The model under review builds one solid part; all positions refer to its coordinate system, in mm. A direction names the side the tool comes from. Coordinates: 2 decimals unless noted, no trailing zeros. Write each loop counter-clockwise with the first axis right and the second up, starting at its lowest first coordinate (ties: lowest second). Pieces come first, ordered by that corner, then holes. Notation, with made-up numbers: (2, -6) -> (11, -6) arc R17 ccw to (11, 9) -> close; hole circle Ø2 at (52.5, -16). An arc over 180 degrees is marked (long way). Put each result on its own line as item: value. Start each with the question number.
from build123d import *

# Parameters (mm, degrees)
BOSS_EXTRUDE1_DEPTH = 50
SKETCH2_R           = 9
CUT_EXTRUDE1_DEPTH  = 50
SKETCH4_R           = 12.5
CUT_EXTRUDE2_DEPTH  = 35
SKETCH7_R           = 35
CUT_EXTRUDE3_DEPTH  = 20
FILLET1_R           = 3
SKETCH8_R           = 50
SKETCH8_R_2         = 43
CUT_EXTRUDE4_DEPTH  = 10
CUT_EXTRUDE5_DEPTH  = 20


with BuildPart() as part:
    # Sketch1 → Boss-Extrude1 (new body)
    with BuildSketch(Plane(origin=(0, 0, 0), x_dir=(1, 0, 0), z_dir=(0, 1, 0))):
        with BuildLine():
            Line((-105, -90), (105, -90))
            ThreePointArc((105, -90), (119.142135624, -84.142135624), (125, -70))
            Line((125, -70), (125, 70))
            ThreePointArc((125, 70), (119.142135624, 84.142135624), (105, 90))
            Line((105, 90), (-105, 90))
            ThreePointArc((-105, 90), (-119.142135624, 84.142135624), (-125, 70))
            Line((-125, 70), (-125, -70))
            ThreePointArc((-125, -70), (-119.142135624, -84.142135624), (-105, -90))
        make_face()
    extrude(amount=BOSS_EXTRUDE1_DEPTH)

    # Sketch2 → Cut-Extrude1 (cut)
    with BuildSketch(Plane(origin=(0, 50, 0), x_dir=(1, 0, 0), z_dir=(0, 1, 0))):
        with Locations((-100, -70)):
            Circle(SKETCH2_R)
        with Locations((-33, -70)):
            Circle(SKETCH2_R)
        with Locations((33, -70)):
            Circle(SKETCH2_R)
        with Locations((100, -70)):
            Circle(SKETCH2_R)
        with Locations((100, 70)):
            Circle(SKETCH2_R)
        with Locations((33, 70)):
            Circle(SKETCH2_R)
        with Locations((-33, 70)):
            Circle(SKETCH2_R)
        with Locations((-100, 70)):
            Circle(SKETCH2_R)
    extrude(amount=-CUT_EXTRUDE1_DEPTH, mode=Mode.SUBTRACT)

    # Sketch4 → Cut-Extrude2 (cut)
    with BuildSketch(Plane(origin=(0, 35, 0), x_dir=(1, 0, 0), z_dir=(0, 1, 0))):
        with Locations((-100, -70)):
            Circle(SKETCH4_R)
        with Locations((-33, -70)):
            Circle(SKETCH4_R)
        with Locations((33, -70)):
            Circle(SKETCH4_R)
        with Locations((100, -70)):
            Circle(SKETCH4_R)
        with Locations((100, 70)):
            Circle(SKETCH4_R)
        with Locations((33, 70)):
            Circle(SKETCH4_R)
        with Locations((-33, 70)):
            Circle(SKETCH4_R)
        with Locations((-100, 70)):
            Circle(SKETCH4_R)
    extrude(amount=-CUT_EXTRUDE2_DEPTH, mode=Mode.SUBTRACT)

    # Sketch7 → Cut-Extrude3 (cut)
    with BuildSketch(Plane(origin=(0, 50, 0), x_dir=(1, 0, 0), z_dir=(0, 1, 0))):
        with Locations((-65, 0)):
            Circle(SKETCH7_R)
        with Locations((65, 0)):
            Circle(SKETCH7_R)
    extrude(amount=-CUT_EXTRUDE3_DEPTH, mode=Mode.SUBTRACT)

    # Fillet1
    fillet1_edges = [part.edges().sort_by_distance(p)[0] for p in [
        (-100, 30, 0),
        (30, 30, 0),
    ]]
    fillet(fillet1_edges, radius=FILLET1_R)

    # Sketch8 → Cut-Extrude4 (cut)
    with BuildSketch(Plane(origin=(0, 50, 0), x_dir=(1, 0, 0), z_dir=(0, 1, 0))):
        with Locations((-65, 0)):
            Circle(SKETCH8_R)
        with Locations((-65, 0)):
            Circle(SKETCH8_R_2, mode=Mode.SUBTRACT)
        with Locations((65, 0)):
            Circle(SKETCH8_R)
        with Locations((65, 0)):
            Circle(SKETCH8_R_2, mode=Mode.SUBTRACT)
    extrude(amount=-CUT_EXTRUDE4_DEPTH, mode=Mode.SUBTRACT)

    # Sketch9 → Cut-Extrude5 (cut)
    with BuildSketch(Plane(origin=(0, 50, 0), x_dir=(1, 0, 0), z_dir=(0, 1, 0))):
        with BuildLine():
            Line((-53.124611797, -79), (-79.875388203, -79))
            ThreePointArc((-79.875388203, -79), (-82.28073938, -77.792842914), (-82.750332745, -75.142857143))
            ThreePointArc((-82.750332745, -75.142857143), (-82.776149203, -64.771332509), (-88.520347372, -56.135744681))
            ThreePointArc((-88.520347372, -56.135744681), (-89.185331801, -52.291224502), (-85.489464765, -51.040981903))
            ThreePointArc((-85.489464765, -51.040981903), (-67.418125523, -54.946816732), (-49.07353502, -52.643591379))
            ThreePointArc((-49.07353502, -52.643591379), (-45.649930196, -53.942627335), (-46.032701785, -57.584337142))
            ThreePointArc((-46.032701785, -57.584337142), (-50.502310556, -65.796534146), (-50.249667255, -75.142857143))
            ThreePointArc((-50.249667255, -75.142857143), (-50.71926062, -77.792842914), (-53.124611797, -79))
        make_face()
        with BuildLine():
            Line((53.124611797, 79), (79.875388203, 79))
            ThreePointArc((79.875388203, 79), (82.28073938, 77.792842914), (82.750332745, 75.142857143))
            ThreePointArc((82.750332745, 75.142857143), (82.776149203, 64.771332509), (88.520347372, 56.135744681))
            ThreePointArc((88.520347372, 56.135744681), (89.185331801, 52.291224502), (85.489464765, 51.040981903))
            ThreePointArc((85.489464765, 51.040981903), (67.418125523, 54.946816732), (49.07353502, 52.643591379))
            ThreePointArc((49.07353502, 52.643591379), (45.649930196, 53.942627335), (46.032701785, 57.584337142))
            ThreePointArc((46.032701785, 57.584337142), (50.502310556, 65.796534146), (50.249667255, 75.142857143))
            ThreePointArc((50.249667255, 75.142857143), (50.71926062, 77.792842914), (53.124611797, 79))
        make_face()
        with BuildLine():
            Line((-53.124611797, 79), (-79.875388203, 79))
            ThreePointArc((-79.875388203, 79), (-82.28073938, 77.792842914), (-82.750332745, 75.142857143))
            ThreePointArc((-82.750332745, 75.142857143), (-82.776149203, 64.771332509), (-88.520347372, 56.135744681))
            ThreePointArc((-88.520347372, 56.135744681), (-89.185331801, 52.291224502), (-85.489464765, 51.040981903))
            ThreePointArc((-85.489464765, 51.040981903), (-67.418125523, 54.946816732), (-49.07353502, 52.643591379))
            ThreePointArc((-49.07353502, 52.643591379), (-45.649930196, 53.942627335), (-46.032701785, 57.584337142))
            ThreePointArc((-46.032701785, 57.584337142), (-50.502310556, 65.796534146), (-50.249667255, 75.142857143))
            ThreePointArc((-50.249667255, 75.142857143), (-50.71926062, 77.792842914), (-53.124611797, 79))
        make_face()
        with BuildLine():
            Line((-12.875388203, -79), (12.875388203, -79))
            ThreePointArc((12.875388203, -79), (15.28073938, -77.792842914), (15.750332745, -75.142857143))
            ThreePointArc((15.750332745, -75.142857143), (18.829727241, -58.900298656), (33.862156902, -52.020659482))
            ThreePointArc((33.862156902, -52.020659482), (36.866627296, -49.927403152), (35.608995423, -46.488373277))
            ThreePointArc((35.608995423, -46.488373277), (10, 0), (35.608995423, 46.488373277))
            ThreePointArc((35.608995423, 46.488373277), (36.866627296, 49.927403152), (33.862156902, 52.020659482))
            ThreePointArc((33.862156902, 52.020659482), (18.829727241, 58.900298656), (15.750332745, 75.142857143))
            ThreePointArc((15.750332745, 75.142857143), (15.28073938, 77.792842914), (12.875388203, 79))
            Line((12.875388203, 79), (-12.875388203, 79))
            ThreePointArc((-12.875388203, 79), (-15.28073938, 77.792842914), (-15.750332745, 75.142857143))
            ThreePointArc((-15.750332745, 75.142857143), (-18.829727241, 58.900298656), (-33.862156902, 52.020659482))
            ThreePointArc((-33.862156902, 52.020659482), (-36.866627296, 49.927403152), (-35.608995423, 46.488373277))
            ThreePointArc((-35.608995423, 46.488373277), (-10, 0), (-35.608995423, -46.488373277))
            ThreePointArc((-35.608995423, -46.488373277), (-36.866627296, -49.927403152), (-33.862156902, -52.020659482))
            ThreePointArc((-33.862156902, -52.020659482), (-18.829727241, -58.900298656), (-15.750332745, -75.142857143))
            ThreePointArc((-15.750332745, -75.142857143), (-15.28073938, -77.792842914), (-12.875388203, -79))
        make_face()
        with BuildLine():
            Line((53.124611797, -79), (79.875388203, -79))
            ThreePointArc((79.875388203, -79), (82.28073938, -77.792842914), (82.750332745, -75.142857143))
            ThreePointArc((82.750332745, -75.142857143), (82.776149203, -64.771332509), (88.520347372, -56.135744681))
            ThreePointArc((88.520347372, -56.135744681), (89.185331801, -52.291224502), (85.489464765, -51.040981903))
            ThreePointArc((85.489464765, -51.040981903), (67.418125523, -54.946816732), (49.07353502, -52.643591379))
            ThreePointArc((49.07353502, -52.643591379), (45.649930196, -53.942627335), (46.032701785, -57.584337142))
            ThreePointArc((46.032701785, -57.584337142), (50.502310556, -65.796534146), (50.249667255, -75.142857143))
            ThreePointArc((50.249667255, -75.142857143), (50.71926062, -77.792842914), (53.124611797, -79))
        make_face()
    extrude(amount=-CUT_EXTRUDE5_DEPTH, mode=Mode.SUBTRACT)


solid = part.part
1. Consider section B-B on x = 2.5. State the section outline as (y, z) points.
2. Insertion check: P1, Ø15, axis at x = -33, z = 70, coming from the -Y side; P2, Ø8.5, axis at x = 70.5, z = -66.5, coming from the +Y side; P3, Ø22.5, axis at x = 100, z = -70, coming from the +Y side; P4, Ø7.5, axis at x = 33.5, z = -64.5, coming from the -Y side. Each pin has a flat end and moves straight along its axis. Give the tip position at first contact, or say it passes through.
3. Consider section D-D on x = 65. State the section outline as (y, z) points, then the cut area to 3 significant figures.
4. Consider section A-A on y = 20. State how many separate pieces and enclosed holes the cut face has, then the cut area to 3 significant figures.
5. Wall thickness on line 1 (Z direction, x = -67, y = 35.5); line 2 (Z direction, x = -65, y = 44.5); line 3 (X direction, y = 44, z = -45.5): over which ranges is each line inside the solid? List them lowest first. Write a range as from..to.
6. Tool access review of faces 1 (the flat face through (0, 40, 79)), 2 (the cylindrical face through (-34.627, 17.745, -82.394)), 3 (the cylindrical face through (31.049, 42.605, -61.214)): name each direction out of +Z, -Z, +X, -X, +Y, -Y from which nothing blocks a thin tool from reaching the whole face with its end or side.
7. The part is to be moulded in two halves that separate along Z. For faces 4 (the cylindrical face through (-119.297, 24.65, 83.986)), 5 (the cylindrical face through (-36.85, 40.14, -49.98)), 6 (the flat face through (-103, 35, 61)), 7 (the flat face through (-30, 50, -41)), say which applies: released by +Z, released by -Z, zero draft, split by the parting line, or undercut.
Output values:
1. outline: (0, -90) -> (50, -90) -> (50, -79) -> (30, -79) -> (30, 79) -> (50, 79) -> (50, 90) -> (0, 90) -> close
2. P1: passes through
2. P2: stops at y = 30
2. P3: stops at y = 50
2. P4: stops at y = 35
3. outline: (0, -90) -> (50, -90) -> (50, -79) -> (30, -79) -> (30, -55) -> (50, -55) -> (50, -50) -> (40, -50) -> (40, -43) -> (50, -43) -> (50, -35) -> (33, -35) arc R3 cw to (30, -32) -> (30, 32) arc R3 cw to (33, 35) -> (50, 35) -> (50, 43) -> (40, 43) -> (40, 50) -> (50, 50) -> (50, 55) -> (30, 55) -> (30, 79) -> (50, 79) -> (50, 90) -> (0, 90) -> close
3. area: 6,500 mm^2
4. separate pieces: 1
4. enclosed holes: 8
4. area: 40,700 mm^2
5. line 1: z = -90..-79, -54.96..-34.94, 34.94..54.96, 79..90
5. line 2: z = -90..-79, -55..-50, -43..-35, 35..43, 50..55, 79..90
5. line 3: x = -125..-85.73, -44.27..-34.1, 34.1..44.27, 85.73..125
6. face 1: +Y
6. face 2: -Y
6. face 3: +Y, -Y
7. face 4: released by +Z
7. face 5: undercut
7. face 6: undercut
7. face 7: zero draft
